from build123d import *

# Parameters (mm, degrees)
SKIZZE1_W                       = 20.3
SKIZZE1_H                       = 20.3
AUFSATZ_LINEAR_AUSTRAGEN1_DEPTH = 10
VERRUNDUNG1_R                   = 0.2
VERRUNDUNG2_R                   = 2.5
SKIZZE2_R                       = 2.3
SCHNITT_LINEAR_AUSTRAGEN1_DEPTH = 40.630953811
FASE2_SIZE                      = 0.5


with BuildPart() as part:
    # Skizze1 → Aufsatz-Linear austragen1 (new body)
    with BuildSketch(Plane.XY):
        with BuildLine():
            Line((14.564597488, 17.15), (-14.564597488, 17.15))
            ThreePointArc((-14.564597488, 17.15), (-15.909902577, 15.909902577), (-17.15, 14.564597488))
            Line((-17.15, 14.564597488), (-17.15, -14.564597488))
            ThreePointArc((-17.15, -14.564597488), (-15.909902577, -15.909902577), (-14.564597488, -17.15))
            Line((-14.564597488, -17.15), (14.564597488, -17.15))
            ThreePointArc((14.564597488, -17.15), (15.909902577, -15.909902577), (17.15, -14.564597488))
            Line((17.15, -14.564597488), (17.15, 14.564597488))
            ThreePointArc((17.15, 14.564597488), (15.909902577, 15.909902577), (14.564597488, 17.15))
        make_face()
        Rectangle(SKIZZE1_W, SKIZZE1_H, mode=Mode.SUBTRACT)
    extrude(amount=AUFSATZ_LINEAR_AUSTRAGEN1_DEPTH)

    # Verrundung1
    verrundung1_edges = [part.edges().sort_by_distance(p)[0] for p in [
        (10.15, -10.15, 5),
        (10.15, 10.15, 5),
        (-10.15, 10.15, 5),
        (-10.15, -10.15, 5),
    ]]
    fillet(verrundung1_edges, radius=VERRUNDUNG1_R)

    # Verrundung2
    verrundung2_edges = [part.edges().sort_by_distance(p)[0] for p in [
        (17.15, 14.564597488, 5),
        (17.15, -14.564597488, 5),
        (14.564597488, -17.15, 5),
        (-14.564597488, -17.15, 5),
        (-17.15, -14.564597488, 5),
        (-17.15, 14.564597488, 5),
        (-14.564597488, 17.15, 5),
        (14.564597488, 17.15, 5),
    ]]
    fillet(verrundung2_edges, radius=VERRUNDUNG2_R)

    # Skizze2 → Schnitt-Linear austragen1 (cut, through all)
    with BuildSketch(Plane(origin=(17.15, 0, 0), x_dir=(0, 0, -1), z_dir=(1, 0, 0))):
        with Locations(Location((-5, 0, 0), (0, 0, 90))):
            Circle(SKIZZE2_R)
    extrude(amount=-SCHNITT_LINEAR_AUSTRAGEN1_DEPTH, mode=Mode.SUBTRACT)

    # Fase2
    fase2_edges = [part.edges().sort_by_distance(p)[0] for p in [
        (-10.15, -2.3, 5),
        (10.15, -2.3, 5),
        (-17.15, -2.3, 5),
        (17.15, -2.3, 5),
        (0, -10.15, 0),
        (0, -10.15, 10),
        (10.15, 0, 0),
        (10.15, 0, 10),
        (-10.15, 0, 0),
        (-10.15, 0, 10),
        (0, 10.15, 0),
        (0, 10.15, 10),
        (10.091421356, -10.091421356, 0),
        (10.091421356, -10.091421356, 10),
        (-10.091421356, -10.091421356, 0),
        (-10.091421356, -10.091421356, 10),
        (-10.091421356, 10.091421356, 0),
        (-10.091421356, 10.091421356, 10),
        (10.091421356, 10.091421356, 0),
        (10.091421356, 10.091421356, 10),
        (0, 17.15, 0),
        (0, 17.15, 10),
        (15.909902577, 15.909902577, 0),
        (17.15, 0, 0),
        (15.909902577, -15.909902577, 0),
        (0, -17.15, 0),
        (-15.909902577, -15.909902577, 0),
        (-17.15, 0, 0),
        (-15.909902577, 15.909902577, 0),
        (-14.52963679, 16.976813809, 0),
        (-16.976813809, 14.52963679, 0),
        (-16.976813809, -14.52963679, 0),
        (-14.52963679, -16.976813809, 0),
        (14.52963679, -16.976813809, 0),
        (16.976813809, -14.52963679, 0),
        (16.976813809, 14.52963679, 0),
        (14.52963679, 16.976813809, 0),
        (15.909902577, 15.909902577, 10),
        (-15.909902577, 15.909902577, 10),
        (-17.15, 0, 10),
        (-15.909902577, -15.909902577, 10),
        (0, -17.15, 10),
        (15.909902577, -15.909902577, 10),
        (17.15, 0, 10),
        (-14.52963679, 16.976813809, 10),
        (-16.976813809, 14.52963679, 10),
        (-16.976813809, -14.52963679, 10),
        (-14.52963679, -16.976813809, 10),
        (14.52963679, -16.976813809, 10),
        (16.976813809, -14.52963679, 10),
        (16.976813809, 14.52963679, 10),
        (14.52963679, 16.976813809, 10),
    ]]
    chamfer(fase2_edges, length=FASE2_SIZE)


solid = part.part
For this review, take the finished solid that the model builds, in its own axes (mm). A direction names the side the tool comes from. Give positions to 0.01 mm unless a question says otherwise; leave off trailing zeros. Write each loop counter-clockwise with the first axis right and the second up, starting at its lowest first coordinate (ties: lowest second). Pieces come first, ordered by that corner, then holes. Notation, with made-up numbers: (9, 33.25) -> (16, 33.25) arc R27 cw to (16, 64.25) -> close; hole circle Ø1 at (9, 48.5). An arc over 180 degrees is marked (long way). Use CSV: the item, a comma, the result in double quotes.
Q1. Take a section at D-D, the plane y = 9. Write out the cut boundary in (x, z).
Conclusion:
outline,"(-17.15, 0.5) -> (-16.65, 0) -> (-10.65, 0) -> (-10.15, 0.5) -> (-10.15, 9.5) -> (-10.65, 10) -> (-16.65, 10) -> (-17.15, 9.5) -> close; (10.15, 0.5) -> (10.65, 0) -> (16.65, 0) -> (17.15, 0.5) -> (17.15, 9.5) -> (16.65, 10) -> (10.65, 10) -> (10.15, 9.5) -> close"
Q2. Tool access review of faces 4 (the face through (-10.15, -2.4, 6.9)), 5 (the face through (16.972, 14.542, 5.063)): name each direction out of +Z, -Z, +X, -X, +Y, -Y from which nothing blocks a thin tool from reaching the whole face with its end or side.
Conclusion:
face 4,"+Z, -Z"
face 5,"+Z, -Z, +X, +Y"
Q3. To check wall thickness, follow probe 1 along Z at (x, y) = (13, 0); probe 2 along Y at (x, z) = (-4.5, 2.75). State the ranges of each line that lie inside material, in increasing order. Write a range as [from, to].
Conclusion:
probe 1,"[0, 2.7], [7.3, 10]"
probe 2,"[-17.15, -10.15], [10.15, 17.15]"
Q4. Mouldability with a two-part tool opening along X and no side actions: class faces 1 (the face through (-16.98, -14.52, 5.06)), 2 (the face through (10.15, -2.4, 6.9)), 3 (the face through (0, 17.15, 5)) as pulls with the +X half, pulls with the -X half, needs draft (parallel to the pull), parting line crosses it, or undercut.
Conclusion:
face 1,"pulls with the -X half"
face 2,"undercut"
face 3,"needs draft"
Q5. Take a section at B-B, the plane z = 1.5. Write out the cut boundary in (x, y).
Conclusion:
outline,"(-17.15, -13.62) arc R2.5 ccw to (-16.48, -15.32) arc R22.5 ccw to (-15.32, -16.48) arc R2.5 ccw to (-13.62, -17.15) -> (13.62, -17.15) arc R2.5 ccw to (15.32, -16.48) arc R22.5 ccw to (16.48, -15.32) arc R2.5 ccw to (17.15, -13.62) -> (17.15, 13.62) arc R2.5 ccw to (16.48, 15.32) arc R22.5 ccw to (15.32, 16.48) arc R2.5 ccw to (13.62, 17.15) -> (-13.62, 17.15) arc R2.5 ccw to (-15.32, 16.48) arc R22.5 ccw to (-16.48, 15.32) arc R2.5 ccw to (-17.15, 13.62) -> close; hole (-10.15, -9.95) arc R0.2 ccw to (-9.95, -10.15) -> (9.95, -10.15) arc R0.2 ccw to (10.15, -9.95) -> (10.15, 9.95) arc R0.2 ccw to (9.95, 10.15) -> (-9.95, 10.15) arc R0.2 ccw to (-10.15, 9.95) -> close"
Q6. Take a section at A-A, the plane y = 0. State how many separate pieces and enclosed holes the cut face has, then the cut area to 3 significant figures.
Conclusion:
separate pieces,"4"
enclosed holes,"0"
area,"73.6 mm2"
Q7. Take a section at C-C, the plane x = 13. Write out the cut boundary in (y, z), then the cut area to 3 significant figures.
Conclusion:
outline,"(-17.15, 0.5) -> (-16.65, 0) -> (16.65, 0) -> (17.15, 0.5) -> (17.15, 9.5) -> (16.65, 10) -> (-16.65, 10) -> (-17.15, 9.5) -> close; hole circle Ø4.6 at (0, 5)"
area,"326 mm2"
